Study the drawing (mm; zero at the part's minimum x, y, z) and answer. A direction names the side the tool comes from. Round coordinates to 2 decimals unless told otherwise and drop trailing zeros. Order: outer loops, then holes, each group sorted by start corner. A loop starts at its lowest first (then second) coordinate and runs counter-clockwise, first axis right, second up. Notation, with made-up numbers: M 45,-21.5 L 62,-21.5 A24 cw 62,6.5 Z; hole C 70,-22 d11. An arc over 180 degrees is marked long. Put each result on its own line as item: value. Start each with the question number.
1. Which of the six approach directions +Z, -Z, +X, -X, +Y, -Y give full straight-line access (tool end or side, diameter ignored) to the marked faces 3, 4 and 5?
2. Consider line 1 (Y direction, x = 78.95, z = 6); line 2 (Y direction, x = 42.1, z = 5.5); line 3 (Y direction, x = 83.5, z = 2.25). Determine where each line is inside the solid, lowest interval first.
3. The part is cut by section A-A (y = 28). Give the vertices of the cut face in (x, z).
4. The part is cut by section D-D (y = 63). Give the vertices of the cut face in (x, z), then the cut area to 4 significant figures.
5. Each of these flat-tipped pins is pushed along its axis until it touches: pin 1 Ø12 at (x, y) = (12, 48) entering from -Z; pin 2 Ø2 at (x, y) = (59.9, 12) entering from -Z. Where does it stop, or does it pass through?
6. The mould has two halves that part along X. Classify the marked faces 1 and 2: +X half, -X half, draft (parallel to the pull), parting line (faces both ways), or undercut.
7. The part is cut by section C-C (x = 42.1). Give the vertices of the cut face in (y, z), then the cut area to 3 significant figures.
8. The part is cut by section B-B (x = 25). Give the vertices of the cut face in (y, z), then the cut area to 3 significant figures.
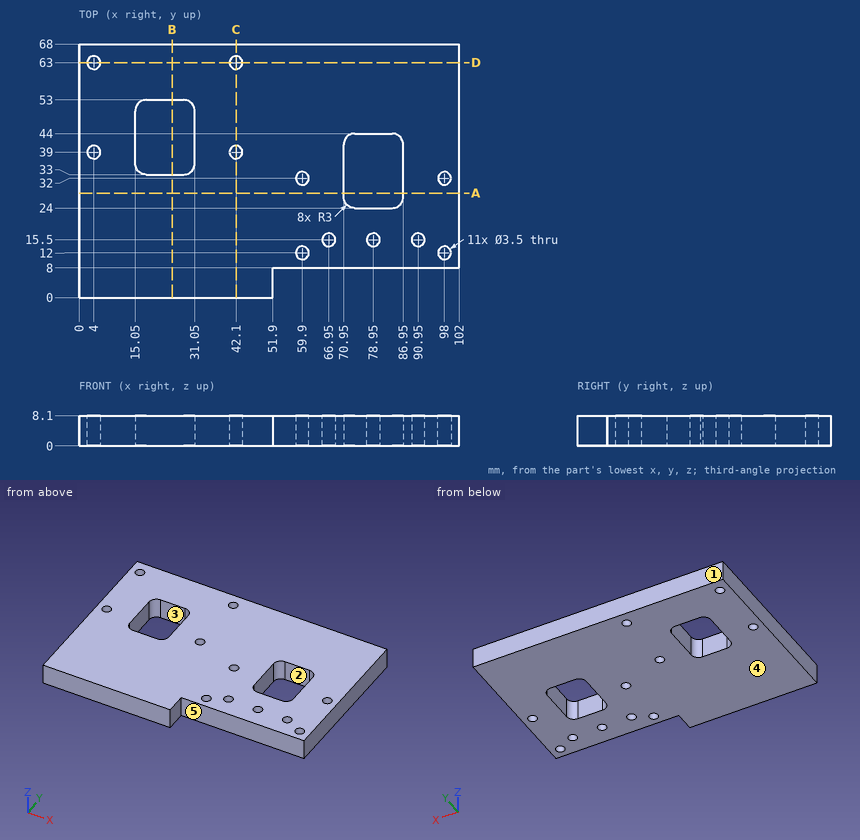
Resolved:
1. face 3: +Z, -Z
1. face 4: -Z, +X, -X, +Y, -Y
1. face 5: +Z, -Z, +X, -Y
2. line 1: 8 to 13.75, 17.25 to 24, 44 to 68
2. line 2: 0 to 37.25, 40.75 to 61.25, 64.75 to 68
2. line 3: 8 to 24, 44 to 68
3. outline: M 0,0 L 70.95,0 L 70.95,8.1 L 0,8.1 Z; M 86.95,0 L 102,0 L 102,8.1 L 86.95,8.1 Z
4. outline: M 0,0 L 2.25,0 L 2.25,8.1 L 0,8.1 Z; M 5.75,0 L 40.35,0 L 40.35,8.1 L 5.75,8.1 Z; M 43.85,0 L 102,0 L 102,8.1 L 43.85,8.1 Z
4. area: 769.5 mm2
5. pin 1: z = 0
5. pin 2: through
6. face 1: draft
6. face 2: undercut
7. outline: M 0,0 L 37.25,0 L 37.25,8.1 L 0,8.1 Z; M 40.75,0 L 61.25,0 L 61.25,8.1 L 40.75,8.1 Z; M 64.75,0 L 68,0 L 68,8.1 L 64.75,8.1 Z
7. area: 494 mm2
8. outline: M 0,0 L 33,0 L 33,8.1 L 0,8.1 Z; M 53,0 L 68,0 L 68,8.1 L 53,8.1 Z
8. area: 389 mm2
